Check sheet for the modelled part. Datum: model origin and axes. Units: mm. A direction names the side the tool comes from. Give positions to 0.01 mm unless a question says otherwise; leave off trailing zeros. Loops run counter-clockwise (first coordinate to the right, second up) from the corner with the lowest first, then second, coordinate; pieces in that order, holes last. Notation, with made-up numbers: M 65,28 L 124,28 A15 ccw 124,56 Z; hole C 72,83.25 d11. An arc over 180 degrees is marked long. Use one line per item in the form item = value.
from build123d import *

# Parameters (mm, degrees)
F1_DEPTH = 10
F2_W     = 20
F2_H     = 10
F3_DEPTH = 10
F5_D     = 6.6


with BuildPart() as f1:
    # F0 (on Top) → F1 (new body)
    with BuildSketch(Plane.XY):
        with BuildLine():
            ThreePointArc((100, 125), (98.5355339059, 128.5355339059), (95, 130))
            Line((95, 130), (-95, 130))
            ThreePointArc((-95, 130), (-98.5355339059, 128.5355339059), (-100, 125))
            Line((-100, 125), (-100, -125))
            ThreePointArc((-100, -125), (-98.5355339059, -128.5355339059), (-95, -130))
            Line((-95, -130), (95, -130))
            ThreePointArc((95, -130), (98.5355339059, -128.5355339059), (100, -125))
            Line((100, -125), (100, 125))
        make_face()
    extrude(amount=F1_DEPTH)

    # F2 (on face) → F3 (cut, through all)
    with BuildSketch(Plane.XY.offset(10)):
        with Locations((-60, -115)):
            Rectangle(F2_W, F2_H)
        with Locations((-20, -115)):
            Rectangle(F2_W, F2_H)
        with Locations((20, -115)):
            Rectangle(F2_W, F2_H)
        with Locations((60, -115)):
            Rectangle(F2_W, F2_H)
        with Locations((60, 115)):
            Rectangle(F2_W, F2_H)
        with Locations((-60, 115)):
            Rectangle(F2_W, F2_H)
        with Locations((20, 115)):
            Rectangle(F2_W, F2_H)
        with Locations((-20, 115)):
            Rectangle(F2_W, F2_H)
    extrude(amount=-F3_DEPTH, mode=Mode.SUBTRACT)

    # F5 (through all)
    with Locations(Plane.XY.offset(10)):
        with Locations((-80, 115), (80, 115), (80, -115), (-80, -115)):
            Hole(F5_D / 2)


solid = f1.part
1) Section check A-A (y = 115). Record the cut outline in (x, z), then the cut area to 3 significant figures.
Evaluation:
outline = M -100,0 L -83.3,0 L -83.3,10 L -100,10 Z; M -76.7,0 L -70,0 L -70,10 L -76.7,10 Z; M -50,0 L -30,0 L -30,10 L -50,10 Z; M -10,0 L 10,0 L 10,10 L -10,10 Z; M 30,0 L 50,0 L 50,10 L 30,10 Z; M 70,0 L 76.7,0 L 76.7,10 L 70,10 Z; M 83.3,0 L 100,0 L 100,10 L 83.3,10 Z
area = 1,070 mm^2
2) Section check C-C (x = -80). Record the cut outline in (y, z), then the cut area to 3 significant figures.
Evaluation:
outline = M -130,0 L -118.3,0 L -118.3,10 L -130,10 Z; M -111.7,0 L 111.7,0 L 111.7,10 L -111.7,10 Z; M 118.3,0 L 130,0 L 130,10 L 118.3,10 Z
area = 2,470 mm^2
3) Depth check by flat-ended pin: pin 1 Ø6 at (x, y) = (-43, 27) entering from -Z. Enter the tip coordinate at first touch or a pass-through.
Evaluation:
pin_1 = 0
4) Release check for a two-part mould opening along Y. For faces 1 (the face through (20, -120, 5)), 2 (the face through (-1, 2, 0)) record: pulls with the +Y half, pulls with the -Y half, needs draft (parallel to the pull), parting line crosses it, or undercut.
Evaluation:
face_1 = undercut
face_2 = needs draft
5) Section check B-B (x = 20). Record the cut outline in (y, z).
Evaluation:
outline = M -130,0 L -120,0 L -120,10 L -130,10 Z; M -110,0 L 110,0 L 110,10 L -110,10 Z; M 120,0 L 130,0 L 130,10 L 120,10 Z
6) Scan lines: line 1 (Y direction, x = -62, z = 8.5); line 2 (Y direction, x = 80, z = 5.5). Record each from-to range of solid material in increasing order.
Evaluation:
line_1 = -130 to -120, -110 to 110, 120 to 130
line_2 = -130 to -118.3, -111.7 to 111.7, 118.3 to 130
7) Set-up check for faces 3 (the face through (-70, 115, 5)), 4 (the face through (-1, 2, 10)): record each of +Z, -Z, +X, -X, +Y, -Y from which the full face is reachable in a straight line by a thin tool's end or side.
Evaluation:
face_3 = +Z, -Z
face_4 = +Z, +X, -X, +Y, -Y
8) Section check D-D (z = 3.75). State how many separate pieces and enclosed holes the cut face has, then the cut area to 3 significant figures.
Evaluation:
separate_pieces = 1
enclosed_holes = 12
area = 50,200 mm^2
